from build123d import *

# Parameters (mm, degrees)
CYLINDER005_R          = 4
CYLINDER005_DEPTH      = 26
CYLINDER005_ROLL_ANGLE = 90
PAD006_DEPTH           = 4


with BuildPart() as cylinder005:
    # Cylinder005 → Cylinder005 (new body)
    with BuildSketch(Plane.XY):
        Circle(CYLINDER005_R)
    extrude(amount=CYLINDER005_DEPTH)


with BuildPart() as cylinder005_1:
    # Cylinder005 roll: moved
    add(cylinder005.part.rotate(Axis((0, 0, 0), (1, 0, 0)), CYLINDER005_ROLL_ANGLE))


with BuildPart() as cylinder005_2:
    # Cylinder005 placement: moved
    add(cylinder005_1.part.moved(Location((4, 1, 6))))


with BuildPart() as basebracket_beveled:
    # Sketch006 → Pad006 (new body)
    with BuildSketch(Plane.XY):
        with BuildLine():
            Line((2.253034, 0.073344), (-63.290852, 0.073344))
            ThreePointArc((-63.290852, 0.073344), (-64.45095, -0.407184), (-64.931478, -1.567282))
            Line((-64.931478, -1.567282), (-64.931478, -11.596925))
            ThreePointArc((-64.931478, -11.596925), (-64.542009, -12.537187), (-63.601747, -12.926656))
            Line((-59.397792, -12.926656), (-63.601747, -12.926656))
            ThreePointArc((-59.397792, -12.926656), (-58.714505, -12.643629), (-58.431478, -11.960342))
            Line((-58.431478, -11.960342), (-58.431478, -6.426656))
            Line((-58.431478, -6.426656), (-2.931478, -6.426656))
            Line((-2.931478, -6.426656), (-2.931478, -17.926656))
            Line((-2.931478, -17.926656), (-8.087364, -17.926656))
            ThreePointArc((-8.087364, -17.926656), (-9.037796, -18.320338), (-9.431478, -19.27077))
            Line((-9.431478, -19.27077), (-9.431478, -23.11525))
            ThreePointArc((-9.431478, -23.11525), (-9.047376, -24.042554), (-8.120072, -24.426656))
            Line((-8.120072, -24.426656), (2.294733, -24.426656))
            ThreePointArc((2.294733, -24.426656), (3.195438, -24.053572), (3.568522, -23.152867))
            Line((3.568522, -1.242144), (3.568522, -23.152867))
            ThreePointArc((3.568522, -1.242144), (3.183225, -0.311953), (2.253034, 0.073344))
        make_face()
    extrude(amount=PAD006_DEPTH)

    # Cut001005: cut Cylinder005
    add(cylinder005_2.part, mode=Mode.SUBTRACT)


solid = basebracket_beveled.part
Design review of the part built by this model. Coordinates are the model's own, in mm. A direction names the side the tool comes from. Round coordinates to 2 decimals unless told otherwise and drop trailing zeros. Write each loop counter-clockwise with the first axis right and the second up, starting at its lowest first coordinate (ties: lowest second). Pieces come first, ordered by that corner, then holes. Notation, with made-up numbers: (-32, 75) - (-2, 75) arc R18 cw to (-2, 89) - close; hole circle Ø1 at (54, 48.25). An arc over 180 degrees is marked (long way). Return JSON: item names as keys, results as strings. Group by question number.
Item 1: For probe 1 along Y at (x, z) = (-7.5, 3.55); probe 2 along Y at (x, z) = (-11, 0.85); probe 3 along X at (y, z) = (-12, 3.65), list the stretches that pass through material, from the lowest coordinate up. Write a range as [from, to].
Item 2: We need section B-B on z = 0.9. Write out the cut boundary in (x, y).
Item 3: We need section D-D on y = -16.25. Write out the cut boundary in (x, z).
Item 4: Machinability: for faces 1 (the face through (-5, -17.927, 2)), 2 (the face through (-61, -12.927, 2)), 3 (the face through (-2.931, -12, 2)), which of the approach directions +Z, -Z, +X, -X, +Y, -Y give a long, thin tool a straight path to every point of the face, cutting with its end or side? Answer none if there is none.
Item 5: We need section C-C on x = -47. Write out the cut boundary in (y, z).
Item 6: We need section A-A on y = -10.75. Write out the cut boundary in (x, z).
Item 7: The part is to be moulded in two halves that separate along X. For faces 4 (the face through (-9.03, -18.31, 1.97)), 5 (the face through (-30, -5, 4)), 6 (the face through (-58.431, -9, 2)), say which applies: pulls with the +X half, pulls with the -X half, needs draft (parallel to the pull), parting line crosses it, or undercut.
Item 8: Insertion check: P1, Ø1.2, axis at y = -10, z = 2.5, coming from the +X side; P2, Ø2, axis at x = -24, z = 1.5, coming from the -Y side; P3, Ø1, axis at y = -12, z = 3.5, coming from the +X side. Each pin has a flat end and moves straight along its axis. Give the tip position at first contact, or say it passes through.
Model answer:
{
 "1": {"probe 1": "y = [-24.43, -17.93], [-6.43, 0.07]", "probe 2": "y = [-6.43, 0.07]", "probe 3": "x = [-64.87, -58.43], [-2.93, 0.76]"},
 "2": {"outline": "(-64.93, -11.6) arc R1.33 ccw to (-63.6, -12.93) - (-59.4, -12.93) arc R0.97 ccw to (-58.43, -11.96) - (-58.43, -6.43) - (-2.93, -6.43) - (-2.93, -17.93) - (-8.09, -17.93) arc R1.34 ccw to (-9.43, -19.27) - (-9.43, -23.12) arc R1.31 ccw to (-8.12, -24.43) - (2.29, -24.43) arc R1.27 ccw to (3.57, -23.15) - (3.57, -1.24) arc R1.32 ccw to (2.25, 0.07) - (-63.29, 0.07) arc R1.64 ccw to (-64.93, -1.57) - close"},
 "3": {"outline": "(-2.93, 0) - (3.57, 0) - (3.57, 2.02) arc R4 cw to (0.54, 4) - (-2.93, 4) - close"},
 "4": {"face 1": "+Z, -Z, -X", "face 2": "+Z, -Z, -X, -Y", "face 3": "+Z, -Z"},
 "5": {"outline": "(-6.43, 0) - (0.07, 0) - (0.07, 4) - (-6.43, 4) - close"},
 "6": {"outline": "(-64.93, 0) - (-58.43, 0) - (-58.43, 4) - (-64.93, 4) - close; (-2.93, 0) - (3.57, 0) - (3.57, 2.02) arc R4 cw to (0.54, 4) - (-2.93, 4) - close"},
 "7": {"face 4": "pulls with the -X half", "face 5": "needs draft", "face 6": "undercut"},
 "8": {"P1": "stops at x = 3.57", "P2": "stops at y = -6.43", "P3": "stops at x = 1.35"}
}
